Can you work these out from the model? Positions are in its coordinate system, mm. Face numbers are marked on the shaded views. Give positions to 0.01 mm unless a question says otherwise; leave off trailing zeros. Order: outer loops, then holes, each group sorted by start corner. A loop starts at its lowest first (then second) coordinate and runs counter-clockwise, first axis right, second up. Notation, with made-up numbers: (8.25, -31.75) - (37.25, -31.75) arc R9 cw to (37.25, -18.75) - close; hole circle Ø1 at (66.5, -36). An arc over 180 degrees is marked (long way). Return JSON: item names as keys, results as strings.
```python
from build123d import *

# Parameters (mm, degrees)
F0_W           = 121
F0_H           = 154
F1_DEPTH       = 10
F2_T           = -2.5
F4_D           = 3
F4_CSINK_D     = 5
F4_CSINK_ANGLE = 90
F5_R           = 1
F6_W           = 10
F6_H           = 5
F7_DEPTH       = 2.5


with BuildPart() as f1:
    # F0 (on Top) → F1 (new body)
    with BuildSketch(Plane.XY):
        with Locations((-30.2418641299, 32.8448046446)):
            Rectangle(F0_W, F0_H)
    extrude(amount=F1_DEPTH)

    # F2
    f2_openings = [f1.faces().sort_by_distance(p)[0] for p in [
        (-30.241864, 32.844805, 10),
    ]]
    offset(amount=F2_T, openings=f2_openings)

    # F4 (through all)
    with Locations(Plane(origin=(0, 0, 0), x_dir=(1, 0, 0), z_dir=(0, 0, -1))):
        with Locations((-80.7418641299, 34.1551953554), (20.2581358701, 34.1551953554), (-80.7418641299, -99.8448046446), (20.2581358701, -99.8448046446)):
            CounterSinkHole(F4_D / 2, F4_CSINK_D / 2, counter_sink_angle=F4_CSINK_ANGLE)

    # F5
    f5_edges = [f1.edges().sort_by_distance(p)[0] for p in [
        (-30.241864, -44.155195, 0),
        (-90.741864, 32.844805, 0),
        (30.258136, 32.844805, 0),
        (-30.241864, 109.844805, 0),
    ]]
    fillet(f5_edges, radius=F5_R)

    # F6 (on face) → F7 (cut, through all)
    with BuildSketch(Plane.XZ.offset(44.1551953554)):
        with Locations((-74.3994042277, 5.5)):
            Rectangle(F6_W, F6_H)
    extrude(amount=-F7_DEPTH, mode=Mode.SUBTRACT)


solid = f1.part
```
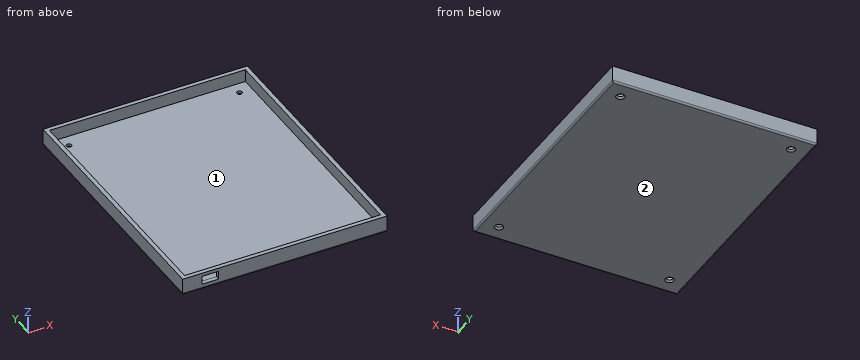
1. Suppose I cut it at B-B (y = 37). List the corners of the cut face in (x, z) for me.
Checks:
{"outline": "(-90.74, 1) arc R1 ccw to (-89.74, 0) - (29.26, 0) arc R1 ccw to (30.26, 1) - (30.26, 10) - (27.76, 10) - (27.76, 2.5) - (-88.24, 2.5) - (-88.24, 10) - (-90.74, 10) - close"}
2. For pin 1 Ø1.8 at (x, y) = (-80.74, 99.84) entering from +Z (3 decimals); pin 2 Ø4 at (x, y) = (20.26, -34.16) entering from +Z, each with a flat end and sliding along its axis, tell me the tip position at first contact or that it passes through.
Checks:
{"pin 1": "through", "pin 2": "z = 2.5"}
3. Suppose I cut it at A-A (x = -76). List the corners of the cut face in (y, z) for me, plus the area to 3 significant figures.
Checks:
{"outline": "(-44.16, 1) arc R1 ccw to (-43.16, 0) - (108.84, 0) arc R1 ccw to (109.84, 1) - (109.84, 10) - (107.34, 10) - (107.34, 2.5) - (-41.66, 2.5) - (-41.66, 3) - (-44.16, 3) - close; (-44.16, 8) - (-41.66, 8) - (-41.66, 10) - (-44.16, 10) - close", "area": "410 mm^2"}
4. Suppose I cut it at D-D (z = 5.5). List the corners of the cut face in (x, y) for me.
Checks:
{"outline": "(-90.74, -44.16) - (-79.4, -44.16) - (-79.4, -41.66) - (-88.24, -41.66) - (-88.24, 107.34) - (27.76, 107.34) - (27.76, -41.66) - (-69.4, -41.66) - (-69.4, -44.16) - (30.26, -44.16) - (30.26, 109.84) - (-90.74, 109.84) - close"}
5. If I drill on L1, parallel to X at y = -23, z = 3; L2, parallel to Y at x = 6.5, z = 3; L3, parallel to Y at x = -73.5, z = 4, over which ranges is the centre line in solid material (lowest first)? Write a range as [from, to].
Checks:
{"L1": "[-90.74, -88.24], [27.76, 30.26]", "L2": "[-44.16, -41.66], [107.34, 109.84]", "L3": "[107.34, 109.84]"}
6. Suppose I cut it at C-C (x = 14). List the corners of the cut face in (y, z) for me, plus the area to 3 significant figures.
Checks:
{"outline": "(-44.16, 1) arc R1 ccw to (-43.16, 0) - (108.84, 0) arc R1 ccw to (109.84, 1) - (109.84, 10) - (107.34, 10) - (107.34, 2.5) - (-41.66, 2.5) - (-41.66, 10) - (-44.16, 10) - close", "area": "422 mm^2"}
7. Thinking about a two-plate mould opening in Y: for the marked faces 1 and 2, which applies, +Y half, -Y half, draft (parallel to the pull), parting line (faces both ways), or undercut?
Checks:
{"face 1": "undercut", "face 2": "draft"}
